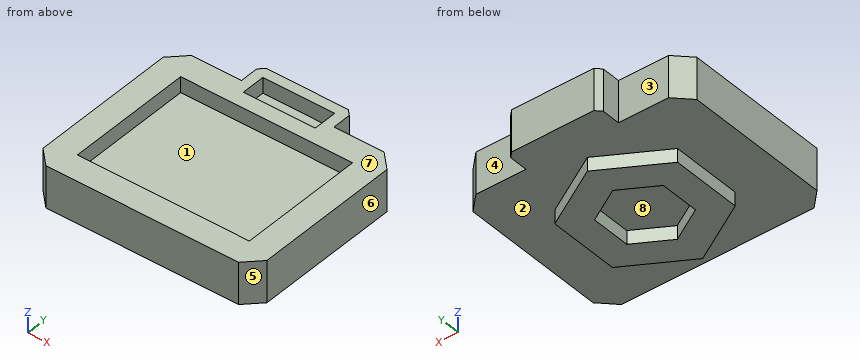
Autodesk Inventor part; units mm, degrees
ref_plane "YZ Plane" through (0, 0, 0) normal (1, 0, 0) x (0, 1, 0)
ref_plane "XZ Plane" through (0, 0, 0) normal (0, 1, 0) x (-1, 0, 0)
ref_plane "XY Plane" through (0, 0, 0) normal (0, 0, 1) x (1, 0, 0)
sketch "Sketch1" plane through (0, 0, 0) normal (0, 0, 1) x (1, 0, 0)
  line L0 (33, 19.0526) -> (33, -19.0526)
  line L1 (33, -19.0526) -> (0, -38.1051)
  line L2 (0, -38.1051) -> (-33, -19.0526)
  line L3 (-33, -19.0526) -> (-33, 19.0526)
  line L4 (-33, 19.0526) -> (0, 38.1051)
  line L5 (0, 38.1051) -> (33, 19.0526)
  line L6 (0, 68.1273) -> (59, 34.0637)
  line L7 (59, 34.0637) -> (59, -34.0637)
  line L8 (59, -34.0637) -> (0, -68.1273)
  line L9 (0, -68.1273) -> (-59, -34.0637)
  line L10 (-59, -34.0637) -> (-59, 34.0637)
  line L11 (-59, 34.0637) -> (0, 68.1273)
  point P0 (0, 0)
  point P1 (0, 0)
  point P2 (0, 0)
  dimension "d0" = 66
  dimension "d1" = 118
extrude "Extrusion1" add sketch "Sketch1" along normal blind 13
sketch "Sketch2" plane through (0, 0, 13) normal (0, 0, 1) x (1, 0, 0)
  line L0 (-82.55, 60.96) -> (82.55, 60.96)
  line L1 (82.55, 60.96) -> (82.55, -60.96)
  line L2 (82.55, -60.96) -> (-82.55, -60.96)
  line L3 (-82.55, -60.96) -> (-82.55, 60.96)
  line L4 (107.55, 85.96) -> (-107.55, 85.96)
  line L5 (-107.55, 85.96) -> (-107.55, -85.96)
  line L6 (-107.55, -85.96) -> (107.55, -85.96)
  line L7 (107.55, -85.96) -> (107.55, 85.96)
  point P0 (0, 0)
  point P1 (0, 60.96)
  point P2 (-82.55, 0)
  dimension "d4" = 165.1
  dimension "d5" = 121.92
  dimension "d6" = 25
extrude "Extrusion2" add sketch "Sketch2" along normal blind 40
sketch "Sketch3" plane through (0, 0, 13) normal (0, 0, 1) x (1, 0, 0)
  line L0 (82.55, 60.96) -> (82.55, -60.96)
  line L1 (82.55, -60.96) -> (-82.55, -60.96)
  line L2 (-82.55, -60.96) -> (-82.55, 60.96)
  line L3 (-82.55, 60.96) -> (82.55, 60.96)
  line L4 (107.55, 85.96) -> (-107.55, 85.96)
  line L5 (-107.55, 85.96) -> (-107.55, -85.96)
  line L6 (-107.55, -85.96) -> (107.55, -85.96)
  line L7 (107.55, -85.96) -> (107.55, 85.96)
  point P0 (0, 0)
extrude "Extrusion3" add sketch "Sketch3" along normal blind 25 contours L0 L1 L2 L3
chamfer "Chamfer1" distance 15 angle 45 4 edges at (107.55, 85.96, 33) (-107.55, 85.96, 33) (-107.55, -85.96, 33) (107.55, -85.96, 33)
sketch "Sketch5" plane through (0, 0, 53) normal (0, 0, 1) x (1, 0, 0)
  line L0 (-34.5, 98.96) -> (34.5, 98.96)
  line L1 (34.5, 98.96) -> (34.5, 75.96)
  line L2 (34.5, 75.96) -> (-34.5, 75.96)
  line L3 (-34.5, 75.96) -> (-34.5, 98.96)
  line L4 (-82.55, 60.96) -> (82.55, 60.96)
  line L5 (-44.5, 65.96) -> (44.5, 65.96)
  line L6 (44.5, 65.96) -> (44.5, 108.96)
  line L7 (44.5, 108.96) -> (-44.5, 108.96)
  line L8 (-44.5, 108.96) -> (-44.5, 65.96)
  point P0 (0, 0)
  point P1 (0, 75.96)
  dimension "d16" = 69
  dimension "d17" = 23
  dimension "d18" = 15
  dimension "d19" = 10
extrude "Extrusion5" cut sketch "Sketch5" against normal through all contours L0 L1 L2 L3
extrude "Extrusion6" add sketch "Sketch5" against normal up to surface (40 mm away) from surface at 0
sketch "Sketch6" plane through (0, 0, 13) normal (0, 0, -1) x (-1, 0, 0)
  line L0 (-34.5, 98.96) -> (34.5, 98.96)
  line L1 (-34.5, 75.96) -> (-34.5, 98.96)
  line L2 (34.5, 98.96) -> (34.5, 75.96)
  line L3 (34.5, 75.96) -> (-34.5, 75.96)
  point P0 (0, 0)
extrude "Extrusion7" add sketch "Sketch6" against normal blind 25
chamfer "Chamfer2" distance 5 angle 45 2 edges at (-44.5, 108.96, 33) (44.5, 108.96, 33)
sketch "Sketch4" plane through (0, 0, 38) normal (0, 0, 1) x (1, 0, 0)
  arc A0 (-11.0008, -6.7698) -> (-71.9286, -8.4622) centre (-38.141, -127.2687) ccw
  arc A1 (-5.9235, 13.5395) -> (-75.3135, 12.2702) centre (-39.1977, -64.7665) ccw
  line L0 (-71.9286, -8.4622) -> (-75.3135, 12.2702)
  line L1 (-5.9235, 13.5395) -> (-11.0008, -6.7698)
  line L2 (0, 0) -> (0, 51.6194) construction
  arc A2 (71.9286, -8.4622) -> (11.0008, -6.7698) centre (38.141, -127.2687) ccw
  arc A3 (75.3135, 12.2702) -> (5.9235, 13.5395) centre (39.1977, -64.7665) ccw
  line L3 (71.9286, -8.4622) -> (75.3135, 12.2702)
  line L4 (5.9235, 13.5395) -> (11.0008, -6.7698)
  arc A4 (-19.0744, -39.0642) -> (63.8895, -28.5788) centre (-4.9616, 182.7337) ccw
  arc A5 (-20.6474, -45.3561) -> (71.9286, -33.1705) centre (-14.0222, 262.0605) ccw
  line L5 (-20.6474, -45.3561) -> (-19.0744, -39.0642)
  line L6 (63.8895, -28.5788) -> (71.9286, -33.1705)
extrude "Extrusion4" [suppressed]
sketch "Sketch7" plane through (0, 0, 38) normal (0, 0, 1) x (1, 0, 0)
  line L0 (-69.7683, 44.5617) -> (-5.8515, 44.5617)
  line L1 (-5.8515, 44.5617) -> (-5.8515, -27.9073)
  line L2 (-5.8515, -27.9073) -> (-69.7683, -27.9073)
  line L3 (-69.7683, -27.9073) -> (-69.7683, 44.5617)
  line L4 (-5.8515, 8.3272) -> (0, 8.3272)
  line L5 (0, 8.3272) -> (0, 0)
  line L6 (0, 0) -> (-5.8515, 0)
  line L7 (-5.8515, 0) -> (-5.8515, 8.3272)
  line L8 (-82.55, -60.96) -> (-82.55, 60.96)
  line L9 (-69.7683, 14.8539) -> (-82.55, 14.8539)
  line L10 (-82.55, 14.8539) -> (-82.55, 4.1636)
  line L11 (-82.55, 4.1636) -> (-69.7683, 4.1636)
  line L12 (-69.7683, 4.1636) -> (-69.7683, 14.8539)
  line L13 (69.7683, 44.5617) -> (5.8515, 44.5617)
  line L14 (5.8515, 44.5617) -> (5.8515, -27.9073)
  line L15 (5.8515, -27.9073) -> (69.7683, -27.9073)
  line L16 (69.7683, -27.9073) -> (69.7683, 44.5617)
  line L17 (5.8515, 8.3272) -> (0, 8.3272)
  line L18 (0, 0) -> (5.8515, 0)
  line L19 (5.8515, 0) -> (5.8515, 8.3272)
  line L20 (82.55, -60.96) -> (82.55, 60.96)
  line L21 (69.7683, 14.8539) -> (82.55, 14.8539)
  line L22 (82.55, 14.8539) -> (82.55, 4.1636)
  line L23 (82.55, 4.1636) -> (69.7683, 4.1636)
  line L24 (69.7683, 4.1636) -> (69.7683, 14.8539)
extrude "Extrusion8" [suppressed]
properties part number "HA11" material "ABS Plastic"
CAD build for the part. Positions are in the model's coordinates, mm. Face numbers are marked on the shaded views. A direction names the side the tool comes from. Give positions to 0.01 mm unless a question says otherwise; leave off trailing zeros. Loops run counter-clockwise (first coordinate to the right, second up) from the corner with the lowest first, then second, coordinate; pieces in that order, holes last. Notation, with made-up numbers: (65, 20.5) - (103, 20.5) arc R7 ccw to (103, 31.5) - close; hole circle Ø1 at (21.25, 28.5). An arc over 180 degrees is marked (long way). Put each result on its own line as item: value.
Q1. Slice it at B-B (z = 21). Give the cut face in (x, y).
Filled in:
outline: (-107.55, -70.96) - (-92.55, -85.96) - (92.55, -85.96) - (107.55, -70.96) - (107.55, 70.96) - (92.55, 85.96) - (44.5, 85.96) - (44.5, 103.96) - (39.5, 108.96) - (-39.5, 108.96) - (-44.5, 103.96) - (-44.5, 85.96) - (-92.55, 85.96) - (-107.55, 70.96) - close
Q2. Mould opens along X. For the marked faces 6, 7 and 8 say: pulls with the +X half, pulls with the -X half, needs draft (parallel to the pull), parting line crosses it, or undercut.
Filled in:
face 6: pulls with the +X half
face 7: needs draft
face 8: undercut
Q3. Slice it at A-A (z = 43). Give the cut face in (x, y).
Filled in:
outline: (-107.55, -70.96) - (-92.55, -85.96) - (92.55, -85.96) - (107.55, -70.96) - (107.55, 70.96) - (92.55, 85.96) - (44.5, 85.96) - (44.5, 103.96) - (39.5, 108.96) - (-39.5, 108.96) - (-44.5, 103.96) - (-44.5, 85.96) - (-92.55, 85.96) - (-107.55, 70.96) - close; hole (-82.55, -60.96) - (82.55, -60.96) - (82.55, 60.96) - (-82.55, 60.96) - close; hole (-34.5, 75.96) - (34.5, 75.96) - (34.5, 98.96) - (-34.5, 98.96) - close
Q4. Slice it at C-C (y = 93). Give the cut face in (x, z), plus the area to 4 significant figures.
Filled in:
outline: (-44.5, 13) - (44.5, 13) - (44.5, 53) - (34.5, 53) - (34.5, 38) - (-34.5, 38) - (-34.5, 53) - (-44.5, 53) - close
area: 2,525 mm²
Q5. Probe line 1 along Y through (x, z) = (64.5, 49.5); line 2 along X through (y, z) = (-4.5, 44.5); line 3 along Z through (x, y) = (-52, 80). List the from-to ranges inside material, lowest first.
Filled in:
line 1: y = -85.96 to -60.96, 60.96 to 85.96
line 2: x = -107.55 to -82.55, 82.55 to 107.55
line 3: z = 13 to 53
Q6. Flat gauge pins, fed straight in: pin 1 (10 mm diameter, centred on x = 1.5, y = -9.5, fed in from -Z); pin 2 (5.5 mm diameter, centred on y = 99, z = 26.5, fed in from -X); pin 3 (20 mm diameter, centred on y = 99.5, z = 24.5, fed in from +X). Where does each tip first touch, or does it go through?
Filled in:
pin 1: stops at z = 13
pin 2: stops at x = -44.5
pin 3: stops at x = 44.5
Q7. Slice it at D-D (x = -62). Give the cut face in (y, z), plus the area to 3 significant figures.
Filled in:
outline: (-85.96, 13) - (85.96, 13) - (85.96, 53) - (60.96, 53) - (60.96, 38) - (-60.96, 38) - (-60.96, 53) - (-85.96, 53) - close
area: 5,050 mm²
Q8. Tool access for the marked faces 1, 2, 3, 4 and 5: list every direction of +Z, -Z, +X, -X, +Y, -Y with a clear straight run to the whole face (end or side of a thin tool).
Filled in:
face 1: +Z
face 2: -Z
face 3: +Z, -Z, -X, +Y
face 4: +Z, -Z, +X, +Y
face 5: +Z, -Z, +X, -Y
